```python
from build123d import *

# Parameters (mm, degrees)
SKETCH1_R           = 6.5
BOSS_EXTRUDE1_DEPTH = 10
SKETCH2_R           = 5
BOSS_EXTRUDE2_DEPTH = 5
SHELL1_T            = -1


with BuildPart() as part:
    # Sketch1 → Boss-Extrude1 (new body)
    with BuildSketch(Plane(origin=(0, 0, 0), x_dir=(1, 0, 0), z_dir=(0, 1, 0))):
        with Locations(Location((0, 0, 0), (0, 0, 270))):
            Circle(SKETCH1_R)
    extrude(amount=BOSS_EXTRUDE1_DEPTH)

    # Sketch2 → Boss-Extrude2 (add)
    with BuildSketch(Plane(origin=(0, 10, 0), x_dir=(1, 0, 0), z_dir=(0, 1, 0))):
        with Locations(Location((0, 0, 0), (0, 0, 270))):
            Circle(SKETCH2_R)
    extrude(amount=BOSS_EXTRUDE2_DEPTH)

    # Shell1
    shell1_openings = [part.faces().sort_by_distance(p)[0] for p in [
        (0, 15, 0),
    ]]
    offset(amount=SHELL1_T, openings=shell1_openings, kind=Kind.INTERSECTION)


solid = part.part
```
Input: part model. Units: mm. Frame: model coordinates. A direction names the side the tool comes from. Round coordinates to 2 decimals unless told otherwise and drop trailing zeros. Loops run counter-clockwise (first coordinate to the right, second up) from the corner with the lowest first, then second, coordinate; pieces in that order, holes last. Notation, with made-up numbers: (47, -27) -> (66, -27) arc R5 cw to (66, -20) -> close; hole circle Ø6 at (81, -28.75). An arc over 180 degrees is marked (long way). Use one line per item in the form item = value. Start each with the question number.
Item 1: Section query C-C on y = 3. Return the cut outline in (x, z).
Item 2: Material intervals for L1, parallel to Y at x = -3.5, z = -3.5; L2, parallel to X at y = 13.65, z = 0; L3, parallel to X at y = 4.75, z = 0, sorted ascending. Write a range as from..to.
Item 3: Mould query, pull axis Y, two halves, no side actions, for faces 1 (the face through (-2, 9, -4)), 2 (the face through (-5, 10, 2)), 3 (the face through (0, 0, 0)). Classes: pulls with the +Y half, pulls with the -Y half, needs draft (parallel to the pull), parting line crosses it, or undercut.
Item 4: Set-up query: faces 4 (the face through (-4.88, 12.46, -1.08)), 5 (the face through (0, 1, 0)), 6 (the face through (-3.955, 4.93, -5.158)). Return all of +Z, -Z, +X, -X, +Y, -Y with unobstructed straight access to the full face (end or side cutting, diameter ignored); none if empty.
Item 5: Section query D-D on x = 4.75. Return the cut outline in (y, z), then the cut area to 3 significant figures.
Item 6: Section query A-A on z = 0. Return the cut outline in (x, y).
Item 7: Contact query for flat-ended pins moving along their axis: pin 1 Ø3 at (y, z) = (6, 2) entering from -X; pin 2 Ø2 at (x, y) = (-2.5, 6) entering from +Z; pin 3 Ø3.5 at (x, z) = (1.5, 0) entering from +Y. Output: stop coordinate, or through.
Item 8: Section query B-B on x = 0. Return the cut outline in (y, z), then the cut area to 3 significant figures.
Ans:
q1.outline = circle Ø13 at (0, 0); hole circle Ø11 at (0, 0)
q2.L1 = 0..1, 9..15
q2.L2 = -5..-4, 4..5
q2.L3 = -6.5..-5.5, 5.5..6.5
q3.face_1 = undercut
q3.face_2 = pulls with the +Y half
q3.face_3 = pulls with the -Y half
q4.face_4 = +Y
q4.face_5 = none
q4.face_6 = +Y, -Y
q5.outline = (0, -4.44) -> (10, -4.44) -> (10, -1.56) -> (15, -1.56) -> (15, 1.56) -> (10, 1.56) -> (10, 4.44) -> (0, 4.44) -> close; hole (1, -2.77) -> (9, -2.77) -> (9, 2.77) -> (1, 2.77) -> close
q5.area = 60.0 mm^2
q6.outline = (-6.5, 0) -> (6.5, 0) -> (6.5, 10) -> (5, 10) -> (5, 15) -> (4, 15) -> (4, 9) -> (5.5, 9) -> (5.5, 1) -> (-5.5, 1) -> (-5.5, 9) -> (-4, 9) -> (-4, 15) -> (-5, 15) -> (-5, 10) -> (-6.5, 10) -> close
q7.pin_1 = -6.48
q7.pin_2 = 6.32
q7.pin_3 = 1
q8.outline = (0, -6.5) -> (10, -6.5) -> (10, -5) -> (15, -5) -> (15, -4) -> (9, -4) -> (9, -5.5) -> (1, -5.5) -> (1, 5.5) -> (9, 5.5) -> (9, 4) -> (15, 4) -> (15, 5) -> (10, 5) -> (10, 6.5) -> (0, 6.5) -> close
q8.area = 44.0 mm^2
